Model file for the job. Use its own axes, mm. Face numbers are marked on the shaded views. A direction names the side the tool comes from. Give positions to 0.01 mm unless a question says otherwise; leave off trailing zeros. Order: outer loops, then holes, each group sorted by start corner. A loop starts at its lowest first (then second) coordinate and runs counter-clockwise, first axis right, second up. Notation, with made-up numbers: (-15.5, 42) -> (1.5, 42) arc R33 ccw to (1.5, 80) -> close; hole circle Ø5 at (56.25, 52.25). An arc over 180 degrees is marked (long way). Answer in a Markdown table with one row per item. Add a question column.
from build123d import *

# Parameters (mm, degrees)
CROQUIS1_W              = 51
CROQUIS1_H              = 17
SALIENTE_EXTRUIR1_DEPTH = 17
CROQUIS2_W              = 15
CROQUIS2_H              = 16
CORTAR_EXTRUIR1_DEPTH   = 17
CROQUIS3_W              = 43
CROQUIS3_H              = 10
CORTAR_EXTRUIR2_DEPTH   = 16
CORTAR_EXTRUIR3_START   = -17
CROQUIS5_R              = 2.55
CORTAR_EXTRUIR3_DEPTH   = 17
CROQUIS6_W              = 49.5
CROQUIS6_H              = 1.4
CORTAR_EXTRUIR4_DEPTH   = 16
CORTAR_EXTRUIR5_START   = -17
CROQUIS7_W              = 6
CROQUIS7_H              = 6
CROQUIS7_W_2            = 20
CROQUIS7_H_2            = 7
CORTAR_EXTRUIR5_DEPTH   = 17
CORTAR_EXTRUIR6_START   = -39
CROQUIS8_W              = 10
CROQUIS8_H              = 6
CORTAR_EXTRUIR6_DEPTH   = 39
CROQUIS10_W             = 17
CROQUIS10_H             = 11
SALIENTE_EXTRUIR4_DEPTH = 1
CROQUIS11_W             = 17
CROQUIS11_H             = 11
SALIENTE_EXTRUIR5_DEPTH = 1
CORTAR_EXTRUIR7_START   = -17
CORTAR_EXTRUIR7_DEPTH   = 17


with BuildPart() as part:
    # Croquis1 → Saliente-Extruir1 (new body)
    with BuildSketch(Plane.XY):
        with Locations((-29.407991935, 18.612308998)):
            Rectangle(CROQUIS1_W, CROQUIS1_H)
    extrude(amount=SALIENTE_EXTRUIR1_DEPTH)

    # Croquis2 → Cortar-Extruir1 (cut)
    with BuildSketch(Plane.XZ.offset(-10.112308998)):
        with Locations((-29.407991935, 9)):
            Rectangle(CROQUIS2_W, CROQUIS2_H)
    extrude(amount=-CORTAR_EXTRUIR1_DEPTH, mode=Mode.SUBTRACT)

    # Croquis3 → Cortar-Extruir2 (cut)
    with BuildSketch(Plane.XY.offset(17)):
        with Locations((-29.407991935, 15.112308998)):
            Rectangle(CROQUIS3_W, CROQUIS3_H)
    extrude(amount=-CORTAR_EXTRUIR2_DEPTH, mode=Mode.SUBTRACT)

    # Croquis5 → Cortar-Extruir3 (cut)
    with BuildSketch(Plane.XY.offset(17).offset(CORTAR_EXTRUIR3_START)):
        with Locations((-43.907991935, 23.612308998)):
            Circle(CROQUIS5_R)
        with Locations((-14.907991935, 23.612308998)):
            Circle(CROQUIS5_R)
    extrude(amount=CORTAR_EXTRUIR3_DEPTH, mode=Mode.SUBTRACT)

    # Croquis6 → Cortar-Extruir4 (cut)
    with BuildSketch(Plane.XY.offset(17)):
        with Locations((-29.407991935, 18.312308998)):
            Rectangle(CROQUIS6_W, CROQUIS6_H)
    extrude(amount=-CORTAR_EXTRUIR4_DEPTH, mode=Mode.SUBTRACT)

    # Croquis7 → Cortar-Extruir5 (cut)
    with BuildSketch(Plane.XY.offset(17).offset(CORTAR_EXTRUIR5_START)):
        with Locations((-6.907991935, 24.112308998)):
            Rectangle(CROQUIS7_W, CROQUIS7_H)
        with Locations((-51.907991935, 24.112308998)):
            Rectangle(CROQUIS7_W, CROQUIS7_H)
        with Locations((-29.407991935, 23.612308998)):
            Rectangle(CROQUIS7_W_2, CROQUIS7_H_2)
    extrude(amount=CORTAR_EXTRUIR5_DEPTH, mode=Mode.SUBTRACT)

    # Croquis8 → Cortar-Extruir6 (cut)
    with BuildSketch(Plane(origin=(-9.907991935, 0, 0), x_dir=(0, 0, -1), z_dir=(1, 0, 0)).offset(CORTAR_EXTRUIR6_START)):
        with Locations((-5, 24.112308998)):
            Rectangle(CROQUIS8_W, CROQUIS8_H)
    extrude(amount=CORTAR_EXTRUIR6_DEPTH, mode=Mode.SUBTRACT)

    # Croquis10 → Saliente-Extruir4 (add)
    with BuildSketch(Plane.ZY.offset(54.907991935)):
        with Locations((8.5, 15.612308998)):
            Rectangle(CROQUIS10_W, CROQUIS10_H)
    extrude(amount=SALIENTE_EXTRUIR4_DEPTH)

    # Croquis11 → Saliente-Extruir5 (add)
    with BuildSketch(Plane(origin=(-3.907991935, 0, 0), x_dir=(0, 0, -1), z_dir=(1, 0, 0))):
        with Locations((-8.5, 15.612308998)):
            Rectangle(CROQUIS11_W, CROQUIS11_H)
    extrude(amount=SALIENTE_EXTRUIR5_DEPTH)

    # Croquis12 → Cortar-Extruir7 (cut)
    with BuildSketch(Plane.XY.offset(17).offset(CORTAR_EXTRUIR7_START)):
        Polygon((-55.907991935, 21.112308998), (-51.907991935, 21.112308998), (-55.907991935, 19.325976361), align=None)
        Polygon((-2.907991935, 21.112308998), (-6.907991935, 21.112308998), (-2.907991935, 19.325976361), align=None)
    extrude(amount=CORTAR_EXTRUIR7_DEPTH, mode=Mode.SUBTRACT)


solid = part.part
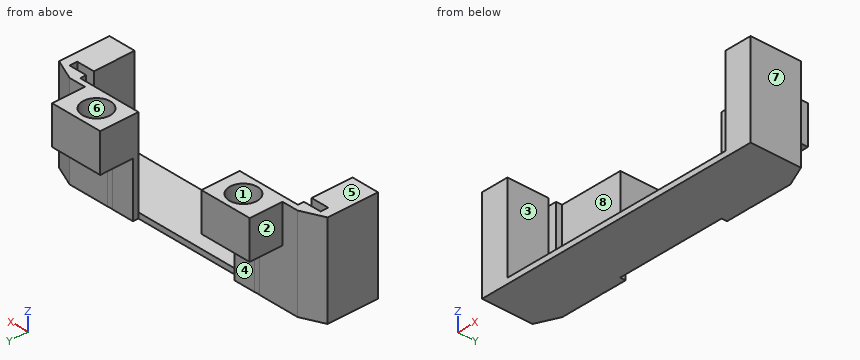
Item 1: Saw through at C-C on z = 12. List the corners of the cut face in (x, y), plus the area to 3 significant figures.
Item 2: Two-plate mould, pull along Y, no slides. Class the marked faces 6, 7 and 8: pulls with the +Y half, pulls with the -Y half, needs draft (parallel to the pull), parting line crosses it, or undercut.
Item 3: Which spindle directions (+Z, -Z, +X, -X, +Y, -Y) get a long thin tool onto all of the face, cutting with end or side? Do the marked faces 1, 2, 3, 4 and 5. Say none if no direction does.
Item 4: Saw through at A-A on z = 7. List the corners of the cut face in (x, y), plus the area to 3 significant figures.
Item 5: Saw through at B-B on y = 15. List the corners of the cut face in (x, z).
Item 6: Saw through at D-D on x = -45. List the corners of the cut face in (y, z).
Item 7: Pin check, flat tips, straight feed: pin 1 Ø2 at (x, z) = (-17.5, 3.5) entering from +Y; pin 2 Ø8 at (x, y) = (-41, 16) entering from +Z; pin 3 Ø3.5 at (x, z) = (-47, 8) entering from -Y; pin 4 Ø3 at (x, y) = (-43.5, 24.5) entering from -Z. Stop position of each tip, or through.
Item 8: Wall check: line 1 (X direction, y = 13.25, z = 15.25); line 2 (Y direction, x = -51, z = 9.25); line 3 (Y direction, x = -39.5, z = 11.5). Give the ranges that are in metal, low to high.
Evaluation:
| question | item | result |
|---|---|---|
| 1 | outline | (-55.91, 10.11) -> (-50.91, 10.11) -> (-50.91, 17.61) -> (-54.16, 17.61) -> (-54.16, 19.01) -> (-50.91, 19.01) -> (-50.91, 20.11) -> (-39.41, 20.11) -> (-39.41, 27.11) -> (-48.91, 27.11) -> (-48.91, 21.11) -> (-51.91, 21.11) -> (-55.91, 19.33) -> close; (-19.41, 20.11) -> (-7.91, 20.11) -> (-7.91, 19.01) -> (-4.66, 19.01) -> (-4.66, 17.61) -> (-7.91, 17.61) -> (-7.91, 10.11) -> (-2.91, 10.11) -> (-2.91, 19.33) -> (-6.91, 21.11) -> (-9.91, 21.11) -> (-9.91, 27.11) -> (-19.41, 27.11) -> close; hole circle Ø5.1 at (-43.91, 23.61); hole circle Ø5.1 at (-14.91, 23.61) |
| 1 | area | 190 mm2 |
| 2 | face 6 | undercut |
| 2 | face 7 | needs draft |
| 2 | face 8 | pulls with the -Y half |
| 3 | face 1 | +Z, -Z |
| 3 | face 2 | +Z, -Z, -X, +Y |
| 3 | face 3 | +Z, -Y |
| 3 | face 4 | -Z, +X, -X, +Y |
| 3 | face 5 | +Z, +X, -X, +Y, -Y |
| 4 | outline | (-55.91, 10.11) -> (-50.91, 10.11) -> (-50.91, 17.61) -> (-54.16, 17.61) -> (-54.16, 19.01) -> (-50.91, 19.01) -> (-50.91, 20.11) -> (-39.41, 20.11) -> (-39.41, 21.11) -> (-43.41, 21.11) arc R2.55 cw to (-44.41, 21.11) -> (-51.91, 21.11) -> (-55.91, 19.33) -> close; (-19.41, 20.11) -> (-7.91, 20.11) -> (-7.91, 19.01) -> (-4.66, 19.01) -> (-4.66, 17.61) -> (-7.91, 17.61) -> (-7.91, 10.11) -> (-2.91, 10.11) -> (-2.91, 19.33) -> (-6.91, 21.11) -> (-14.41, 21.11) arc R2.55 cw to (-15.41, 21.11) -> (-19.41, 21.11) -> close |
| 4 | area | 117 mm2 |
| 5 | outline | (-55.91, 0) -> (-2.91, 0) -> (-2.91, 17) -> (-7.91, 17) -> (-7.91, 1) -> (-50.91, 1) -> (-50.91, 17) -> (-55.91, 17) -> close |
| 6 | outline | (10.11, 0) -> (21.11, 0) -> (21.11, 10) -> (21.31, 10) -> (21.31, 17) -> (20.11, 17) -> (20.11, 1) -> (10.11, 1) -> close; (25.92, 10) -> (27.11, 10) -> (27.11, 17) -> (25.92, 17) -> close |
| 7 | pin 1 | stops at y = 21.11 |
| 7 | pin 2 | stops at z = 1 |
| 7 | pin 3 | stops at y = 20.11 |
| 7 | pin 4 | passes through |
| 8 | line 1 | x = -55.91 to -50.91, -7.91 to -2.91 |
| 8 | line 2 | y = 10.11 to 17.61, 19.01 to 21.11 |
| 8 | line 3 | y = 20.11 to 27.11 |
